from build123d import *

# Parameters (mm, degrees)
SKETCH2_W           = 50
SKETCH2_H           = 65
BOSS_EXTRUDE1_DEPTH = 12
BOSS_EXTRUDE2_DEPTH = 12
SKETCH5_R           = 12.5
CUT_EXTRUDE1_DEPTH  = 12
SKETCH7_W           = 12
SKETCH7_H           = 30
BOSS_EXTRUDE3_DEPTH = 25


with BuildPart() as part:
    # Sketch2 → Boss-Extrude1 (new body)
    with BuildSketch(Plane(origin=(0, 0, 0), x_dir=(1, 0, 0), z_dir=(0, 1, 0))):
        with Locations((25, -32.5)):
            Rectangle(SKETCH2_W, SKETCH2_H)
    extrude(amount=BOSS_EXTRUDE1_DEPTH)

    # Sketch3 → Boss-Extrude2 (add)
    with BuildSketch(Plane(origin=(0, 12, 0), x_dir=(1, 0, 0), z_dir=(0, 1, 0))):
        with BuildLine():
            Line((0, -65), (50, -65))
            ThreePointArc((50, -65), (25, -90), (0, -65))
        make_face()
    extrude(amount=-BOSS_EXTRUDE2_DEPTH)

    # Sketch5 → Cut-Extrude1 (cut)
    with BuildSketch(Plane(origin=(0, 12, 0), x_dir=(1, 0, 0), z_dir=(0, 1, 0))):
        with Locations(Location((25, -65, 0), (0, 0, 270))):
            Circle(SKETCH5_R)
    extrude(amount=-CUT_EXTRUDE1_DEPTH, mode=Mode.SUBTRACT)

    # Sketch7 → Boss-Extrude3 (add)
    with BuildSketch(Plane(origin=(0, 12, 0), x_dir=(1, 0, 0), z_dir=(0, 1, 0))):
        with Locations((44, -15)):
            Rectangle(SKETCH7_W, SKETCH7_H)
    extrude(amount=BOSS_EXTRUDE3_DEPTH)


solid = part.part
Verification items for the finished model (mm, model axes). A direction names the side the tool comes from. Coordinates: 2 decimals unless noted, no trailing zeros. Order: outer loops, then holes, each group sorted by start corner. A loop starts at its lowest first (then second) coordinate and runs counter-clockwise, first axis right, second up. Notation, with made-up numbers: (65, 33.5) -> (100, 33.5) arc R15 cw to (100, 57.5) -> close; hole circle Ø7 at (-15, 40). An arc over 180 degrees is marked (long way). Put each result on its own line as item: value. Start each with the question number.
1. Cross-section at B-B, the plane y = 9. Record the boundary of the cut face in (x, z).
2. Mould release check, pull along Z, two halves, no side actions. Record for faces 1 (the flat face through (0, 6, 33)), 2 (the cylindrical face through (12.797, 6.084, 62.29)), 3 (the flat face through (30, 10, 0)): released by +Z, released by -Z, zero draft, split by the parting line, or undercut.
3. Material ranges on L1, parallel to X at y = 8.25, z = 65; L2, parallel to Z at x = 42, y = 23.5; L3, parallel to Y at x = 15.5, z = 84.5, recorded low to high. Write a range as [from, to].
4. Cross-section at A-A, the plane x = 25. Record the boundary of the cut face in (y, z), then the cut area to 3 significant figures.
5. Cross-section at D-D, the plane y = 34. Record the boundary of the cut face in (x, z), then the cut area to 3 significant figures.
6. Go/stop test with flat-tipped pins: pin 1 Ø20 at (y, z) = (25.5, 10.5) entering from -X; pin 2 Ø22.5 at (x, z) = (25, 65) entering from +Y; pin 3 Ø3.5 at (x, y) = (41.5, 19) entering from +Z; pin 4 Ø25 at (x, z) = (22, 40) entering from +Y. Record where each tip stops, or that it passes through.
7. Access from +Z, -Z, +X, -X, +Y, -Y to the whole of each face (thin tool, end or side, straight path). Record for faces 4 (the flat face through (44, 24, 30)), 5 (the flat face through (38, 24, 15)), 6 (the cylindrical face through (25.55, 6.084, 89.994)).
8. Cross-section at C-C, the plane x = 14. Record the boundary of the cut face in (y, z), then the cut area to 3 significant figures.
Computed:
1. outline: (0, 0) -> (50, 0) -> (50, 65) arc R25 ccw to (0, 65) -> close; hole circle Ø25 at (25, 65)
2. face 1: zero draft
2. face 2: undercut
2. face 3: released by -Z
3. L1: [0, 12.5], [37.5, 50]
3. L2: [0, 30]
3. L3: [0, 12]
4. outline: (0, 0) -> (12, 0) -> (12, 52.5) -> (0, 52.5) -> close; (0, 77.5) -> (12, 77.5) -> (12, 90) -> (0, 90) -> close
4. area: 780 mm2
5. outline: (38, 0) -> (50, 0) -> (50, 30) -> (38, 30) -> close
5. area: 360 mm2
6. pin 1: x = 38
6. pin 2: through
6. pin 3: z = 30
6. pin 4: y = 12
7. face 4: +Z, +X, -X, +Y
7. face 5: +Z, -Z, -X, +Y
7. face 6: +Z, +Y, -Y
8. outline: (0, 0) -> (12, 0) -> (12, 59.06) -> (0, 59.06) -> close; (0, 70.94) -> (12, 70.94) -> (12, 87.45) -> (0, 87.45) -> close
8. area: 907 mm2
